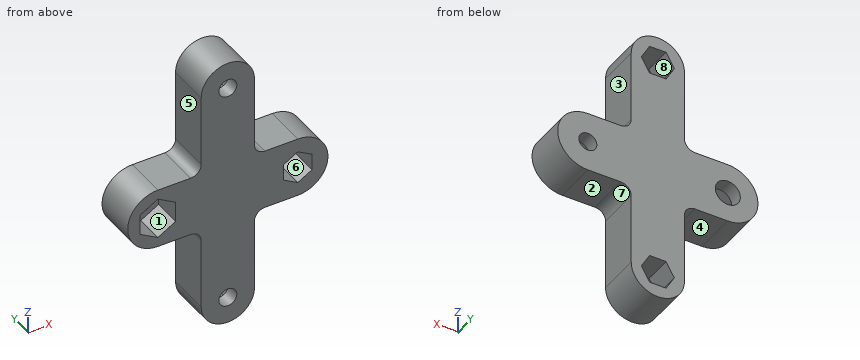
Autodesk Inventor part; units mm, degrees
ref_plane "YZ Plane" through (0, 0, 0) normal (1, 0, 0) x (0, 1, 0)
ref_plane "XZ Plane" through (0, 0, 0) normal (0, 1, 0) x (-1, 0, 0)
ref_plane "XY Plane" through (0, 0, 0) normal (0, 0, 1) x (1, 0, 0)
sketch "Sketch1" plane through (0, 0, 0) normal (0, 1, 0) x (-1, 0, 0)
  circle A0 centre (0, 0) radius 2.55
  circle A1 centre (0, -63.56) radius 2.55
  line L0 (0, 0) -> (0, -63.56) construction
  line L1 (0, 0) -> (0, -63.56) construction
  line L2 (-7.55, 0) -> (-7.55, -20.23)
  line L3 (7.55, -63.56) -> (7.55, -43.33)
  arc A2 (7.55, 0) -> (-7.55, 0) centre (0, 0) ccw
  arc A3 (-7.55, -63.56) -> (7.55, -63.56) centre (0, -63.56) ccw
  line L4 (19.85, -31.78) -> (-19.85, -31.78) construction
  circle A4 centre (19.85, -31.78) radius 3.55
  circle A5 centre (-19.85, -31.78) radius 2.55
  line L5 (19.85, -31.78) -> (-19.85, -31.78) construction
  line L6 (19.85, -23.23) -> (10.55, -23.23)
  line L7 (-19.85, -40.33) -> (-10.55, -40.33)
  arc A6 (19.85, -40.33) -> (19.85, -23.23) centre (19.85, -31.78) ccw
  arc A7 (-19.85, -23.23) -> (-19.85, -40.33) centre (-19.85, -31.78) ccw
  line L8 (7.55, -40.33) -> (7.55, -23.23) construction
  line L9 (-7.55, -43.33) -> (-7.55, -63.56)
  line L10 (-7.55, -23.23) -> (-7.55, -40.33) construction
  line L11 (7.55, -20.23) -> (7.55, 0)
  line L12 (7.55, -23.23) -> (-7.55, -23.23) construction
  line L13 (-10.55, -23.23) -> (-19.85, -23.23)
  line L14 (10.55, -40.33) -> (19.85, -40.33)
  line L15 (-7.55, -40.33) -> (7.55, -40.33) construction
  arc A8 (7.55, -20.23) -> (10.55, -23.23) centre (10.55, -20.23) ccw
  arc A9 (-10.55, -23.23) -> (-7.55, -20.23) centre (-10.55, -20.23) ccw
  arc A10 (-7.55, -43.33) -> (-10.55, -40.33) centre (-10.55, -43.33) ccw
  arc A11 (10.55, -40.33) -> (7.55, -43.33) centre (10.55, -43.33) ccw
  point P0 (0, -31.78)
  point P1 (0, -31.78)
  point P2 (0, -31.78)
  dimension "d0" = 5.1
  dimension "d1" = 5.1
  dimension "d2" = 63.56
  dimension "d3" = 5
  dimension "d18" = 39.7
  dimension "d19" = 7.1
  dimension "d20" = 5.1
  dimension "d22" = 3
  dimension "d31" = 5
extrude "Extrusion1" add sketch "Sketch1" along normal blind 12
sketch "Sketch5" plane through (0, 12, 0) normal (0, 1, 0) x (1, 0, 0)
  line L0 (2.3383, 4.05) -> (4.6765, 0)
  line L1 (4.6765, 0) -> (2.3383, -4.05)
  line L2 (2.3383, -4.05) -> (-2.3383, -4.05)
  line L3 (-2.3383, -4.05) -> (-4.6765, 0)
  line L4 (-4.6765, 0) -> (-2.3383, 4.05)
  line L5 (-2.3383, 4.05) -> (2.3383, 4.05)
  circle A0 centre (0, 63.56) radius 2.55
  line L6 (-2.3383, 59.51) -> (-4.6765, 63.56)
  line L7 (-4.6765, 63.56) -> (-2.3383, 67.61)
  line L8 (-2.3383, 67.61) -> (2.3383, 67.61)
  line L9 (2.3383, 67.61) -> (4.6765, 63.56)
  line L10 (4.6765, 63.56) -> (2.3383, 59.51)
  line L11 (2.3383, 59.51) -> (-2.3383, 59.51)
  point P0 (0, 0)
  point P1 (0, 0)
  dimension "d23" = 8.1
  dimension "d24" = 8.1
extrude "Extrusion4" cut sketch "Sketch5" against normal blind 8 contours L0 L1 L2 L3 L4 L5 | A0 | L6 L7 L8 L9 L10 L11
sketch "Sketch6" plane through (0, 0, 0) normal (0, -1, 0) x (1, 0, 0)
  circle A0 centre (-19.85, -31.78) radius 3.55
  line L0 (-14.8, -28.8644) -> (-14.8, -34.6956)
  line L1 (-14.8, -34.6956) -> (-19.85, -37.6112)
  line L2 (-19.85, -37.6112) -> (-24.9, -34.6956)
  line L3 (-24.9, -34.6956) -> (-24.9, -28.8644)
  line L4 (-24.9, -28.8644) -> (-19.85, -25.9488)
  line L5 (-19.85, -25.9488) -> (-14.8, -28.8644)
  circle A1 centre (19.85, -31.78) radius 2.55
  line L6 (15.8, -34.1183) -> (15.8, -29.4417)
  line L7 (15.8, -29.4417) -> (19.85, -27.1035)
  line L8 (19.85, -27.1035) -> (23.9, -29.4417)
  line L9 (23.9, -29.4417) -> (23.9, -34.1183)
  line L10 (23.9, -34.1183) -> (19.85, -36.4565)
  line L11 (19.85, -36.4565) -> (15.8, -34.1183)
  point P0 (0, 0)
  dimension "d27" = 10.1
  dimension "d28" = 8.1
extrude "Extrusion5" cut sketch "Sketch6" against normal blind 8
properties part number "Acoplador" material "ABS Plastic"
The listing builds one solid part. Answer for the finished solid, in the listing's coordinates (mm). Face numbers are marked on the shaded views. A direction names the side the tool comes from. Coordinates: 2 decimals unless noted, no trailing zeros. Loops run counter-clockwise (first coordinate to the right, second up) from the corner with the lowest first, then second, coordinate; pieces in that order, holes last. Notation, with made-up numbers: (-28.75, 51.5) -> (18.25, 51.5) arc R12 cw to (18.25, 73.5) -> close; hole circle Ø2 at (72, 26). An arc over 180 degrees is marked (long way). Answer in a Markdown table with one row per item. Add a question column.
1. The part is cut by section B-B, the plane x = 0. Write down the section's boundary in (y, z), then the cut area to 3 significant figures.
2. Determine the mould class of the marked faces 5, 6, 7 and 8 for opening direction Z: +Z half, -Z half, draft (parallel to the pull), parting line (faces both ways), or undercut.
3. Consider line 1 (X direction, y = 10.75, z = -31.78); line 2 (Z direction, x = 0, y = 2); line 3 (Z direction, x = -0.5, y = 9). Determine where each line is inside the solid, lowest interval first. Write a range as [from, to].
4. The part is cut by section A-A, the plane y = 10. Count the separate pieces of the cut face and the enclosed holes in it, then the cut area to 3 significant figures.
5. The part is cut by section C-C, the plane z = -5. Write down the section's boundary in (x, y), then the cut area to 3 significant figures.
6. For the marked faces 1, 2, 3 and 4, determine the directions among +Z, -Z, +X, -X, +Y, -Y from which every point of the face is accessible in a straight line to the end or side of a thin tool.
7. Flat-ended cylindrical pins translate along their axes: P1, Ø6, axis at x = -9, z = -40, coming from the -Y side; P2, Ø3, axis at x = 17, y = 3, coming from the +Z side; P3, Ø1.5, axis at x = 14.5, y = 1.5, coming from the -Z side; P4, Ø6.5, axis at x = 0, z = 0.5, coming from the +Y side. Find the tip coordinate at first contact, or state that the pin passes through.
8. The part is cut by section D-D, the plane x = 12. Write down the section's boundary in (y, z).
Answer below:
| question | item | result |
|---|---|---|
| 1 | outline | (0, -71.11) -> (12, -71.11) -> (12, -67.61) -> (4, -67.61) -> (4, -66.11) -> (0, -66.11) -> close; (0, -61.01) -> (4, -61.01) -> (4, -59.51) -> (12, -59.51) -> (12, -4.05) -> (4, -4.05) -> (4, -2.55) -> (0, -2.55) -> close; (0, 2.55) -> (4, 2.55) -> (4, 4.05) -> (12, 4.05) -> (12, 7.55) -> (0, 7.55) -> close |
| 1 | area | 774 mm2 |
| 2 | face 5 | draft |
| 2 | face 6 | undercut |
| 2 | face 7 | -Z half |
| 2 | face 8 | undercut |
| 3 | line 1 | [-28.4, -23.4], [-16.3, 17.3], [22.4, 28.4] |
| 3 | line 2 | [-71.11, -66.11], [-61.01, -2.55], [2.55, 7.55] |
| 3 | line 3 | [-71.09, -67.61], [-59.51, -4.05], [4.05, 7.53] |
| 4 | separate pieces | 1 |
| 4 | enclosed holes | 4 |
| 4 | area | 1,620 mm2 |
| 5 | outline | (-7.55, 0) -> (7.55, 0) -> (7.55, 12) -> (-7.55, 12) -> close |
| 5 | area | 181 mm2 |
| 6 | face 1 | -Y |
| 6 | face 2 | -Z, +X, +Y, -Y |
| 6 | face 3 | +Z, +X, +Y, -Y |
| 6 | face 4 | -Z, -X, +Y, -Y |
| 7 | P1 | y = 0 |
| 7 | P2 | z = -23.23 |
| 7 | P3 | z = -40.33 |
| 7 | P4 | y = 4 |
| 8 | outline | (0, -40.33) -> (12, -40.33) -> (12, -23.23) -> (0, -23.23) -> close |
